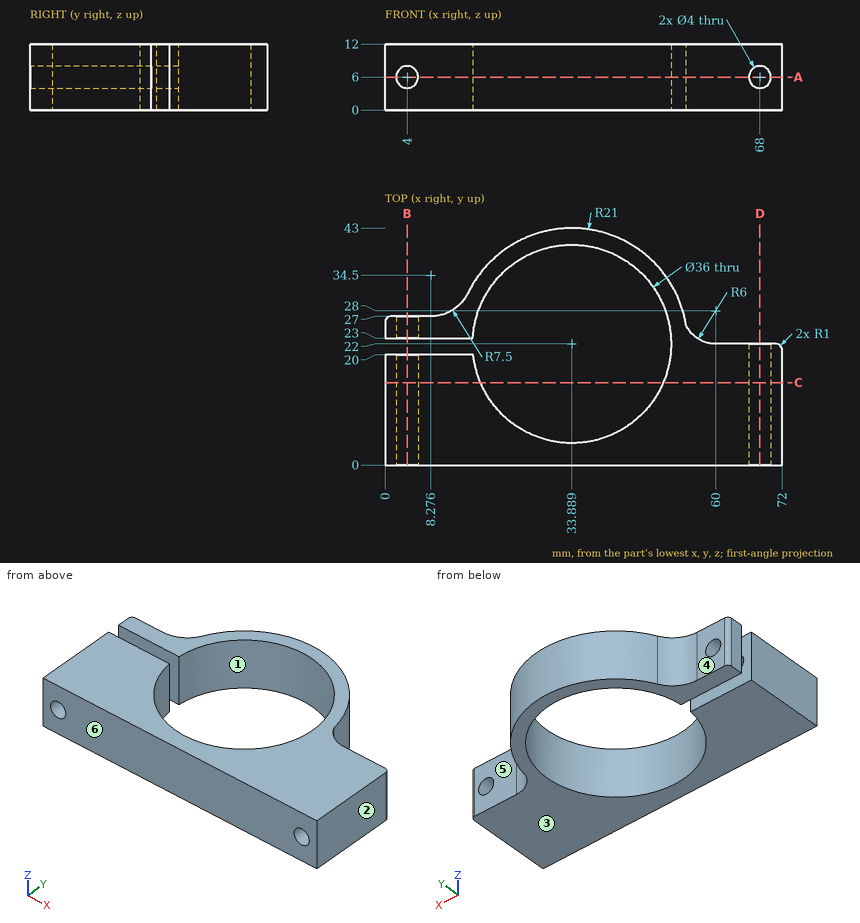
Print and shaded views of the part. All mm, measured from the part's lowest x, y and z. A direction names the side the tool comes from. Round coordinates to 2 decimals unless told otherwise and drop trailing zeros. Write each loop counter-clockwise with the first axis right and the second up, starting at its lowest first coordinate (ties: lowest second). Pieces come first, ordered by that corner, then holes. Notation, with made-up numbers: M 48,-3 L 100,-3 A23 cw 100,33 Z; hole C -29,-37.75 d9. An arc over 180 degrees is marked long. Use a Markdown table: item, result. Add a question column.
1. Slice it at B-B on x = 4. Give the cut face in (y, z).
2. Drill centre lines: probe 1 along Y at (x, z) = (7, 3.25); probe 2 along X at (y, z) = (25.5, 5.5) (1 decimal); probe 3 along Y at (x, z) = (69.5, 0.75). Where is each one in solid material? Low to high.
3. 3-axis set-ups, long thin cutter, end or side, ignore diameter. For the marked faces 4, 5 and 6: which of +Z, -Z, +X, -X, +Y, -Y reach the whole face in a straight line?
4. Slice it at A-A on z = 6. Give the cut face in (x, y), then the cut area to 3 significant figures.
5. Slice it at C-C on y = 15. Give the cut face in (x, z) (1 decimal).
6. Pull direction X, two halves, no side cores. Call the marked faces 1, 2 and 3: released by +X, released by -X, zero draft, split by the parting line, or undercut.
7. Flat gauge pins, fed straight in: P1, Ø5, axis at x = 10, z = 5.5, coming from the +Y side; P2, Ø5, axis at x = 4, z = 6, coming from the +Y side; P3, Ø4.5, axis at x = 68, z = 6, coming from the +Y side; P4, Ø2.5, axis at x = 4, z = 6, coming from the +Y side. Where does each tip first touch, or does it go through?
8. Slice it at D-D on x = 68. Give the cut face in (y, z).
Reply:
| question | item | result |
|---|---|---|
| 1 | outline | M 0,0 L 20,0 L 20,4 L 0,4 Z; M 0,8 L 20,8 L 20,12 L 0,12 Z; M 23,0 L 27,0 L 27,4 L 23,4 Z; M 23,8 L 27,8 L 27,12 L 23,12 Z |
| 2 | probe 1 | y = 0 to 20, 23 to 27 |
| 2 | probe 2 | x = 0 to 2.1, 5.9 to 16.2, 51.5 to 54.6 |
| 2 | probe 3 | y = 0 to 22 |
| 3 | face 4 | +Z, -Z, -X, +Y |
| 3 | face 5 | +Z, -Z, +X, +Y |
| 3 | face 6 | +Z, -Z, +X, -X, -Y |
| 4 | outline | M 0,0 L 2,0 L 2,20 L 0,20 Z; M 0,23 L 2,23 L 2,27 L 1,27 A1 ccw 0,26 Z; M 6,0 L 66,0 L 66,22 L 60,22 A6 cw 54.62,25.34 A21 ccw 15.02,31.21 A7.5 cw 8.28,27 L 6,27 L 6,23 L 15.92,23 A18 cw long 16,20 L 6,20 Z; M 70,0 L 72,0 L 72,21 A1 ccw 71,22 L 70,22 Z |
| 4 | area | 1,100 mm^2 |
| 5 | outline | M 0,0 L 17.3,0 L 17.3,12 L 0,12 Z; M 50.5,0 L 72,0 L 72,12 L 50.5,12 Z; hole C 4,6 d4; hole C 68,6 d4 |
| 6 | face 1 | undercut |
| 6 | face 2 | released by +X |
| 6 | face 3 | zero draft |
| 7 | P1 | stops at y = 28.3 |
| 7 | P2 | stops at y = 27 |
| 7 | P3 | stops at y = 22 |
| 7 | P4 | passes through |
| 8 | outline | M 0,0 L 22,0 L 22,4 L 0,4 Z; M 0,8 L 22,8 L 22,12 L 0,12 Z |
